```python
from build123d import *

# Parameters (mm, degrees)
SKETCH1_R           = 25
BOSS_EXTRUDE1_DEPTH = 315.095017
SKETCH2_R           = 19.079270484
CUT_EXTRUDE1_DEPTH  = 318.07234149
CHAMFER1_SIZE       = 4.06661
CHAMFER1_SIZE_2     = 7.043576


with BuildPart() as part:
    # Sketch1 → Boss-Extrude1 (new body)
    with BuildSketch(Plane(origin=(0, 0, 0), x_dir=(1, 0, 0), z_dir=(0, 1, 0))):
        with Locations(Location((0, 0, 0), (0, 0, 270))):
            Circle(SKETCH1_R)
    extrude(amount=BOSS_EXTRUDE1_DEPTH)

    # Sketch2 → Cut-Extrude1 (cut, through all)
    with BuildSketch(Plane(origin=(0, 0, 0), x_dir=(1, 0, 0), z_dir=(0, 1, 0))):
        with Locations(Location((0, 0, 0), (0, 0, 270))):
            Circle(SKETCH2_R)
    extrude(amount=CUT_EXTRUDE1_DEPTH, mode=Mode.SUBTRACT)

    # Chamfer1
    # the kernel refuses this chamfer: 7.043576, 4.06661 mm, written as the material it takes off along each edge
    with BuildSketch(Plane(origin=(0, 315.095017, 0), x_dir=(0, 0, 1), z_dir=(-1, 0, 0))) as chamfer1_piece_1:
        Polygon((25, -CHAMFER1_SIZE), (25 - CHAMFER1_SIZE_2, 0), (25, 0), align=None)
    revolve(axis=Axis((0, 315.095017, 0), (0, 1, 0)), mode=Mode.SUBTRACT)
    with BuildSketch(Plane(origin=(0, 0, 0), x_dir=(0, 0, 1), z_dir=(-1, 0, 0))) as chamfer1_piece_2:
        Polygon((25, CHAMFER1_SIZE_2), (25 - CHAMFER1_SIZE, 0), (25, 0), align=None)
    revolve(axis=Axis((0, 0, 0), (0, 1, 0)), mode=Mode.SUBTRACT)


solid = part.part
```
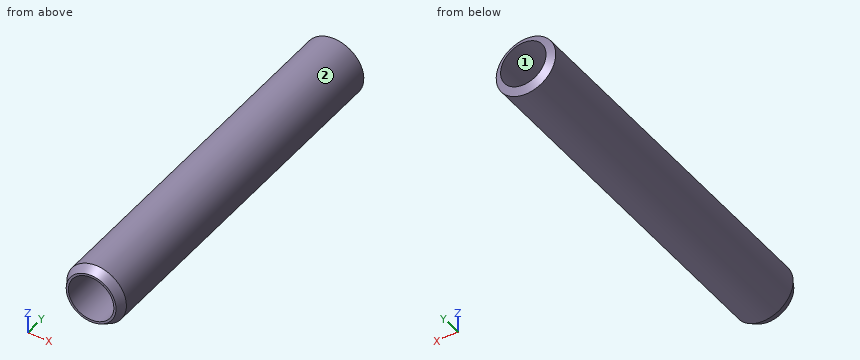
Can you work these out from the model? Positions are in its coordinate system, mm. Face numbers are marked on the shaded views. Round coordinates to 2 decimals unless told otherwise and drop trailing zeros. Loops run counter-clockwise (first coordinate to the right, second up) from the corner with the lowest first, then second, coordinate; pieces in that order, holes last.
Item 1: Please list where these lines run through material, in increasing order: L1, parallel to X at y = 113, z = 0; L2, parallel to X at y = 190.5, z = -8; L3, parallel to Z at x = -3.5, y = 94.5.
Item 2: Suppose I cut it at A-A, the plane z = 0. Write out the boundary of the cut face in (x, y).
Item 3: If we mould it in two halves opening along X, with no side actions, what happens to the marked faces 1 and 2? For each: +X half, -X half, draft (parallel to the pull), parting line (faces both ways), or undercut.
Item 4: Suppose I cut it at C-C, the plane y = 205. Write out the boundary of the cut face in (x, z).
Item 5: Suppose I cut it at B-B, the plane x = 0. Write out the boundary of the cut face in (y, z), then the cut area to 3 significant figures.
Item 6: Will these pins go through, and if not, where does the flat tip stop? pin 1 Ø6 at (x, y) = (4.5, 246.5) entering from -Z; pin 2 Ø2 at (y, z) = (88.5, 9.5) entering from -X; pin 3 Ø12 at (x, y) = (-19.5, 171) entering from -Z; pin 4 Ø12 at (x, z) = (-1.5, 10.5) entering from -Y.
Reported:
1. L1: x = -25 to -19.08, 19.08 to 25
1. L2: x = -23.69 to -17.32, 17.32 to 23.69
1. L3: z = -24.75 to -18.76, 18.76 to 24.75
2. outline: (-25, 7.04) - (-20.93, 0) - (-19.08, 0) - (-19.08, 314.45) - (-25, 311.03) - close; (19.08, 0) - (20.93, 0) - (25, 7.04) - (25, 311.03) - (19.08, 314.45) - close
3. face 1: undercut
3. face 2: parting line
4. outline: circle Ø50 at (0, 0); hole circle Ø38.16 at (0, 0)
5. outline: (0, -20.93) - (7.04, -25) - (311.03, -25) - (314.45, -19.08) - (0, -19.08) - close; (0, 19.08) - (314.45, 19.08) - (311.03, 25) - (7.04, 25) - (0, 20.93) - close
5. area: 3,670 mm2
6. pin 1: stops at z = -24.95
6. pin 2: stops at x = -23.51
6. pin 3: stops at z = -21.04
6. pin 4: passes through
